from build123d import *

# Parameters (mm, degrees)
BOSS_EXTRUDE1_DEPTH = 40
SKETCH2_W           = 21
SKETCH2_H           = 43
CUT_EXTRUDE1_DEPTH  = 80
CUT_EXTRUDE2_DEPTH  = 80
SKETCH4_W           = 34
SKETCH4_H           = 18
BOSS_EXTRUDE3_DEPTH = 52
CUT_EXTRUDE3_DEPTH  = 13
HOLE1_D             = 20
FILLET1_R           = 8


with BuildPart() as part:
    # Sketch1 → Boss-Extrude1 (new, symmetric)
    with BuildSketch(Plane(origin=(0, 0, 0), x_dir=(0, 0, -1), z_dir=(1, 0, 0))):
        Polygon((0, 0), (0, 40), (52, 40), (52, 61), (70, 61), (70, 25), (22, 25), (22, 0), align=None)
    extrude(amount=BOSS_EXTRUDE1_DEPTH, both=True)

    # Sketch2 → Cut-Extrude1 (cut)
    with BuildSketch(Plane.XY):
        with Locations((-29.5, 39.5)):
            Rectangle(SKETCH2_W, SKETCH2_H)
        with Locations((29.5, 39.5)):
            Rectangle(SKETCH2_W, SKETCH2_H)
    extrude(amount=-CUT_EXTRUDE1_DEPTH, mode=Mode.SUBTRACT)

    # Sketch3 → Cut-Extrude2 (cut)
    with BuildSketch(Plane.XY):
        Polygon((25, 18), (40, 10), (40, 18), align=None)
    cut_extrude2 = extrude(amount=-CUT_EXTRUDE2_DEPTH, mode=Mode.SUBTRACT)

    # Mirror1: Cut-Extrude2 across plane
    add(cut_extrude2.mirror(Plane(origin=(0, 0, 0), x_dir=(0, 0, 1), z_dir=(1, 0, 0))), mode=Mode.SUBTRACT)

    # Sketch4 → Boss-Extrude3 (add)
    with BuildSketch(Plane.XY):
        with Locations((0, 9)):
            Rectangle(SKETCH4_W, SKETCH4_H)
    extrude(amount=BOSS_EXTRUDE3_DEPTH)

    # Sketch5 → Cut-Extrude3 (cut)
    with BuildSketch(Plane(origin=(0, 18, 0), x_dir=(1, 0, 0), z_dir=(0, 1, 0))):
        with BuildLine():
            Line((-10, -27), (-10, -52))
            Line((-10, -52), (10, -52))
            Line((10, -52), (10, -27))
            ThreePointArc((10, -27), (0, -17), (-10, -27))
        make_face()
    extrude(amount=-CUT_EXTRUDE3_DEPTH, mode=Mode.SUBTRACT)

    # Sketch6 → Revolve1 (revolve)
    with BuildSketch(Plane(origin=(0, 61, 0), x_dir=(1, 0, 0), z_dir=(0, 1, 0))):
        Polygon((6, 52), (10, 70), (12, 70), (8, 52), align=None)
    revolve(axis=Axis((0, 61, 0), (0, 0, -1)))

    # Hole1 (through all)
    with Locations(Plane(origin=(0, 40, 0), x_dir=(1, 0, 0), z_dir=(0, 1, 0))):
        with Locations((0, 32)):
            Hole(HOLE1_D / 2)

    # Fillet1
    fillet1_edges = [part.edges().sort_by_distance(p)[0] for p in [
        (0, 40, 0),
    ]]
    fillet(fillet1_edges, radius=FILLET1_R)


solid = part.part
Model file for the job. Use its own axes, mm. A direction names the side the tool comes from. Give positions to 0.01 mm unless a question says otherwise; leave off trailing zeros. Write each loop counter-clockwise with the first axis right and the second up, starting at its lowest first coordinate (ties: lowest second). Pieces come first, ordered by that corner, then holes. Notation, with made-up numbers: (27, 11.5) -> (44, 11.5) arc R12 cw to (44, 32.5) -> close; hole circle Ø10 at (66, 40). An arc over 180 degrees is marked (long way). Write item = value, one per line.
(1) Tool access for faces 1 (the face through (-22, 18, -11)), 2 (the face through (17, 9, 26)), 3 (the face through (-17, 9, 26)): list every direction of +Z, -Z, +X, -X, +Y, -Y with a clear straight run to the whole face (end or side of a thin tool).
Determined:
face_1 = +Z, -Z, -X, +Y
face_2 = +Z, +X, +Y, -Y
face_3 = +Z, -X, +Y, -Y
(2) Slice it at B-B, the plane y = 30.5. Give the cut face in (x, z), then the cut area to 3 significant figures.
Determined:
outline = (-19, -70) -> (19, -70) -> (19, 0) -> (-19, 0) -> close; hole circle Ø20 at (0, -32)
area = 2,350 mm2
(3) Slice it at C-C, the plane z = 41.5. Give the cut face in (x, y), then the cut area to 3 significant figures.
Determined:
outline = (-17, 0) -> (17, 0) -> (17, 18) -> (10, 18) -> (10, 5) -> (-10, 5) -> (-10, 18) -> (-17, 18) -> close
area = 352 mm2
(4) Probe line 1 along Z through (x, y) = (0, 29); line 2 along X through (y, z) = (59, -55.5); line 3 along X through (y, z) = (32.5, -35). List the from-to ranges inside material, lowest first.
Determined:
line_1 = -70 to -42, -22 to 0
line_2 = -19 to 19
line_3 = -19 to -9.54, 9.54 to 19
(5) Slice it at A-A, the plane z = -32. Give the cut face in (x, y), then the cut area to 3 significant figures.
Determined:
outline = (-19, 25) -> (-10, 25) -> (-10, 40) -> (-19, 40) -> close; (10, 25) -> (19, 25) -> (19, 40) -> (10, 40) -> close
area = 270 mm2
(6) Slice it at D-D, the plane x = -15.5. Give the cut face in (y, z), then the cut area to 3 significant figures.
Determined:
outline = (0, -22) -> (25, -22) -> (25, -70) -> (61, -70) -> (61, -52) -> (40, -52) -> (40, -8) arc R8 ccw to (32, 0) -> (18, 0) -> (18, 52) -> (0, 52) -> close
area = 2,900 mm2
(7) Mould opens along X. For faces 4 (the face through (0, 69, -61)), 5 (the face through (0, 5, 34)), 6 (the face through (-32.39, 14.06, -10.85)), 7 (the face through (0, 3, 52)) say: released by +X, released by -X, zero draft, split by the parting line, or undercut.
Determined:
face_4 = undercut
face_5 = undercut
face_6 = released by -X
face_7 = zero draft
(8) Flat gauge pins, fed straight in: P1, Ø14.5, axis at y = 11.5, z = 31.5, coming from the +X side; P2, Ø4, axis at y = 8.5, z = 34, coming from the -X side; P3, Ø5, axis at x = 23.5, z = -8.5, coming from the +Y side; P4, Ø12, axis at y = 49.5, z = -33.5, coming from the -X side. Where does each tip first touch, or does it go through?
Determined:
P1 = 17
P2 = -17
P3 = 18
P4 = through
